Geometry: final body of the model. Coordinates: model frame, mm. Give positions to 0.01 mm unless a question says otherwise; leave off trailing zeros. Loops run counter-clockwise (first coordinate to the right, second up) from the corner with the lowest first, then second, coordinate; pieces in that order, holes last.
1. Material intervals for line 1 along Z through (x, y) = (0, 8.5); line 2 along X through (y, z) = (2.5, -0.25); line 3 along X through (y, z) = (5, -0.25), sorted ascending.
2. Section D-D, the plane z = -1.25. Output: boundary loops of the cut face in (x, y), then the cut area to 3 significant figures.
3. Section C-C, the plane z = 0.5. Output: boundary loops of the cut face in (x, y).
4. Section A-A, the plane x = 0. Output: boundary loops of the cut face in (y, z).
5. Draft query along X for faces 1 (the face through (4, -4, 5)), 2 (the face through (-0.54, 7.13, -2.44)), 3 (the face through (-1.08, -4.88, -0.06)), 4 (the face through (-2.17, -9.76, 0.06)). Return one class per face: +X half, -X half, draft (parallel to the pull), parting line (faces both ways), or undercut.
6. Section B-B, the plane z = -3.25. Output: boundary loops of the cut face in (x, y).
7. First-contact query: P1, Ø1, axis at y = -1.5, z = 3.5, coming from the +X side; P2, Ø3, axis at y = -8, z = -1.5, coming from the -X side; P3, Ø3, axis at x = 0, z = 0, coming from the +Y side. Flat tips, straight axial feed; report the tip coordinate or a pass-through.
from build123d import *

# Parameters (mm, degrees)
SKETCH_R     = 10
SKETCH_R_2   = 5
PAD_DEPTH    = 5
SKETCH001_R  = 2.5
POCKET_DEPTH = 10.001
CHAMFER_SIZE = 0.5


with BuildPart() as part:
    # Sketch → Pad (new body, symmetric)
    with BuildSketch(Plane.XY):
        Circle(SKETCH_R)
        Circle(SKETCH_R_2, mode=Mode.SUBTRACT)
    extrude(amount=PAD_DEPTH, both=True)

    # Sketch001 → Pocket (cut, through all)
    with BuildSketch(Plane.XZ):
        Circle(SKETCH001_R)
    extrude(amount=-POCKET_DEPTH, mode=Mode.SUBTRACT)

    # Chamfer
    chamfer_edges = [part.edges().sort_by_distance(p)[0] for p in [
        (-5, 0, -5),
        (-10, 0, -5),
        (-5, 0, 5),
        (-10, 0, 5),
    ]]
    chamfer(chamfer_edges, length=CHAMFER_SIZE)


solid = part.part
Answers below:
1. line 1: z = -5 to -2.5, 2.5 to 5
1. line 2: x = -9.68 to -4.33, 4.33 to 9.68
1. line 3: x = -8.66 to -2.49, 2.49 to 8.66
2. outline: (-2.17, 4.51) - (-2.17, 9.76) arc R10 ccw (long way) to (2.17, 9.76) - (2.17, 4.51) arc R5 cw (long way) to start
2. area: 214 mm2
3. outline: (-2.45, 4.36) - (-2.45, 9.7) arc R10 ccw (long way) to (2.45, 9.7) - (2.45, 4.36) arc R5 cw (long way) to start
4. outline: (-10, -4.5) - (-9.5, -5) - (-5.5, -5) - (-5, -4.5) - (-5, 4.5) - (-5.5, 5) - (-9.5, 5) - (-10, 4.5) - close; (5, -4.5) - (5.5, -5) - (9.5, -5) - (10, -4.5) - (10, -2.5) - (5, -2.5) - close; (5, 2.5) - (10, 2.5) - (10, 4.5) - (9.5, 5) - (5.5, 5) - (5, 4.5) - close
5. face 1: draft
5. face 2: undercut
5. face 3: undercut
5. face 4: parting line
6. outline: circle Ø20 at (0, 0); hole circle Ø10 at (0, 0)
7. P1: stops at x = 9.95
7. P2: stops at x = -7.6
7. P3: stops at y = -4.77
